```python
from build123d import *

# Parameters (mm, degrees)
F1_DEPTH = 127
F2_W     = 101.6
F2_H     = 76.2
F3_DEPTH = 6.35
F4_W     = 76.2
F4_H     = 6.35
F5_DEPTH = 25.4
F7_DEPTH = 6.35
F8_R     = 3.17499
F9_R     = 3.17499


# Not quite as in the source:
# - a fillet or chamfer is up to 0.001 mm smaller than in the source, because OpenCascade refuses the exact size


with BuildPart() as f1:
    # F0 (on Right) → F1 (new body)
    with BuildSketch(Plane.YZ):
        Polygon((-65.1389909149, 110.2977480159), (-82.7816457659, 10.2412803099), (120.4183542341, 10.2412803099), (120.4183542341, 162.6412803099), align=None)
    extrude(amount=F1_DEPTH)

    # F2 (on face) → F3 (cut)
    with BuildSketch(Plane(origin=(0, -82.036835794, 14.4653075624), x_dir=(1, 0, 0), z_dir=(0, -0.984807753, 0.1736481777))):
        with Locations((63.5, 46.5108103184)):
            Rectangle(F2_W, F2_H)
    extrude(amount=-F3_DEPTH, mode=Mode.SUBTRACT)

    # F4 (on face) → F5 (cut)
    with BuildSketch(Plane(origin=(0, -33.6216432412, 119.1884190074), x_dir=(1, 0, 0), z_dir=(0, -0.2714930529, 0.9624403993))):
        with Locations((63.5, 21.2276759098)):
            Rectangle(F4_W, F4_H)
    extrude(amount=-F5_DEPTH, mode=Mode.SUBTRACT)

    # F6 (on face) → F7 (join)
    with BuildSketch(Plane(origin=(0, -33.6216432412, 119.1884190074), x_dir=(1, 0, 0), z_dir=(0, -0.2714930529, 0.9624403993))):
        Polygon((25.4, 30.7526759098), (25.4, 24.4026759098), (101.6, 24.4026759098), (101.6, 18.0526759098), (101.6, 11.7026759098), (107.95, 11.7026759098), (107.95, 30.7526759098), align=None)
        Polygon((25.4, 18.0526759098), (25.4, 24.4026759098), (25.4, 30.7526759098), (19.05, 30.7526759098), (19.05, 11.7026759098), (101.6, 11.7026759098), (101.6, 18.0526759098), align=None)
    extrude(amount=F7_DEPTH)

    # F8 (radius 3.175 in the source; OpenCascade refuses exactly that, so slightly less here)
    f8_edges = [f1.edges().sort_by_distance(p)[0] for p in [
        (63.5, -22.358515, 122.365614),
        (107.95, -13.19127, 124.951586),
        (63.5, -4.024026, 127.537557),
        (19.05, -13.19127, 124.951586),
        (63.5, -24.082496, 128.477111),
        (107.95, -14.915251, 131.063082),
        (63.5, -5.748006, 133.649053),
        (19.05, -14.915251, 131.063082),
        (19.05, -23.220506, 125.421362),
        (19.05, -4.886016, 130.593305),
        (107.95, -23.220506, 125.421362),
        (107.95, -4.886016, 130.593305),
        (63.5, -11.859503, 131.925073),
        (101.6, -14.915251, 131.063082),
        (63.5, -17.971, 130.201092),
        (25.4, -14.915251, 131.063082),
        (25.4, -13.661047, 114.92235),
        (25.4, -7.549551, 116.646331),
        (101.6, -7.549551, 116.646331),
        (101.6, -13.661047, 114.92235),
    ]]
    fillet(f8_edges, radius=F8_R)

    # F9 (radius 3.175 in the source; OpenCascade refuses exactly that, so slightly less here)
    f9_edges = [f1.edges().sort_by_distance(p)[0] for p in [
        (63.5, -3.239599, 101.36759),
    ]]
    fillet(f9_edges, radius=F9_R)


solid = f1.part
```
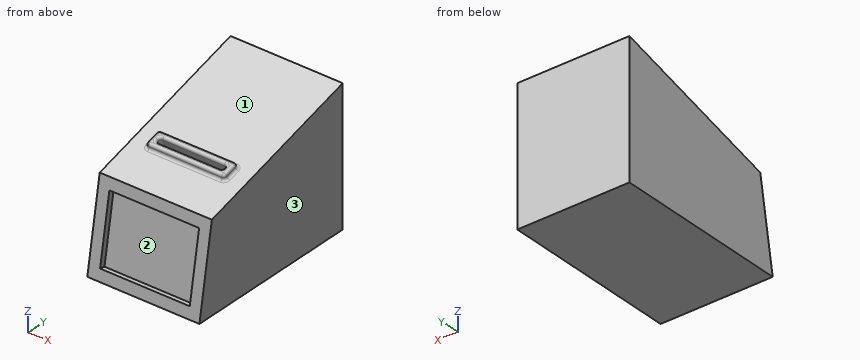
Model file for the job. Use its own axes, mm. Face numbers are marked on the shaded views. Give positions to 0.01 mm unless a question says otherwise; leave off trailing zeros. Write each loop counter-clockwise with the first axis right and the second up, starting at its lowest first coordinate (ties: lowest second). Pieces come first, ordered by that corner, then holes. Notation, with made-up numbers: (22, 56) -> (43, 56) arc R12 ccw to (43, 77) -> close; hole circle Ø6 at (77, 53.5). An arc over 180 degrees is marked (long way). Use CSV: the item, a comma, the result in double quotes. Start each with the question number.
1) Two-plate mould, pull along X, no slides. Class the marked faces 1, 2 and 3: released by +X, released by -X, zero draft, split by the parting line, or undercut.
2) Cut at C-C on y = 27. List the corners of the cut face in (x, z).
3) Drill centre lines: L1, parallel to Y at x = 67, z = 123; L2, parallel to Z at x = 116, y = -25.5; L3, parallel to Z at x = 74.5, y = -30. Where is each one in solid material? Low to high.
4) Cut at D-D on z = 66. List the corners of the cut face in (x, y).
5) Cut at B-B on z = 25.5. List the corners of the cut face in (x, y).
6) Pin check, flat tips, straight feed: P1, Ø5, axis at x = 54.5, z = 34.5, coming from the -Y side; P2, Ø5, axis at x = 49.5, y = -31.5, coming from the +Z side; P3, Ø1.7, axis at y = -16, z = 127.5, coming from the +X side (3 decimals). Stop position of each tip, or through.
Final values:
1,face 1,"zero draft"
1,face 2,"undercut"
1,face 3,"released by +X"
2,outline,"(0, 10.24) -> (127, 10.24) -> (127, 136.29) -> (0, 136.29) -> close"
3,L1,"y = -23.51 to -15.94, -9.34 to 120.42"
3,L2,"z = 10.24 to 121.48"
3,L3,"z = 10.24 to 120.21"
4,outline,"(0, -72.95) -> (12.7, -72.95) -> (12.7, -66.5) -> (114.3, -66.5) -> (114.3, -72.95) -> (127, -72.95) -> (127, 120.42) -> (0, 120.42) -> close"
5,outline,"(0, -80.09) -> (12.7, -80.09) -> (12.7, -73.64) -> (114.3, -73.64) -> (114.3, -80.09) -> (127, -80.09) -> (127, 120.42) -> (0, 120.42) -> close"
6,P1,"stops at y = -72.5"
6,P2,"stops at z = 120.49"
6,P3,"stops at x = 108.055"
